from build123d import *

# Parameters (mm, degrees)
F1_DEPTH  = 25.4
F2_R      = 5.08
F3_T      = -6.35
F4_R      = 3.175
F5_DEPTH  = 38.1
F8_DEPTH  = 87.2033022895
F9_R      = 3.175
F10_DEPTH = 87.2033022895
F11_R     = 2.54
F12_DEPTH = 38.1


# Not quite as in the source:
# - the program builds the solid bodies; features that only make, move or delete a surface that nothing else refers to are left out


with BuildPart() as f1:
    # F0 (on Top) → F1 (new body)
    with BuildSketch(Plane.XY):
        Polygon((-43.9940905122, -76.2), (43.9940905122, -76.2), (87.9881810245, 0), (43.9940905122, 76.2), (-43.9940905122, 76.2), (-87.9881810245, 0), align=None)
    extrude(amount=F1_DEPTH)

    # F2
    f2_edges = [f1.edges().sort_by_distance(p)[0] for p in [
        (-65.991136, -38.1, 25.4),
        (0, -76.2, 25.4),
        (65.991136, -38.1, 25.4),
        (65.991136, 38.1, 25.4),
        (0, 76.2, 25.4),
        (-65.991136, 38.1, 25.4),
        (43.994091, -76.2, 12.7),
        (87.988181, 0, 12.7),
        (-43.994091, -76.2, 12.7),
        (43.994091, 76.2, 12.7),
        (-43.994091, 76.2, 12.7),
        (-87.988181, 0, 12.7),
    ]]
    fillet(f2_edges, radius=F2_R)

    # F3
    f3_openings = [f1.faces().sort_by_distance(p)[0] for p in [
        (0, 0, 0),
    ]]
    offset(amount=F3_T, openings=f3_openings)

    # F4 (on Right) → F5 (join)
    with BuildSketch(Plane.YZ):
        with Locations((76.2, 0)):
            Circle(F4_R)
    extrude(amount=-F5_DEPTH)

    # F8 (cut, through all): a face of the model
    f8_faces = [f1.faces().sort_by_distance(p)[0] for p in [
        (0, 76.6491706172, -0.4491706172),
    ]]
    extrude(f8_faces, amount=F8_DEPTH, mode=Mode.SUBTRACT)

    # F9 (on face) → F10 (cut, through all)
    with BuildSketch(Plane.YZ):
        with Locations((76.2, 0)):
            Circle(F9_R)
    extrude(amount=F10_DEPTH, mode=Mode.SUBTRACT)

    # F11 (on face) → F12 (join)
    with BuildSketch(Plane.YZ):
        with Locations((76.2, 0)):
            Circle(F11_R)
    extrude(amount=F12_DEPTH)


solid = f1.part
The listing builds one solid part. Answer for the finished solid, in the listing's coordinates (mm). A direction names the side the tool comes from. Coordinates: 2 decimals unless noted, no trailing zeros. Write each loop counter-clockwise with the first axis right and the second up, starting at its lowest first coordinate (ties: lowest second). Pieces come first, ordered by that corner, then holes. Notation, with made-up numbers: (63.5, 21) - (70.5, 21) arc R15 ccw to (70.5, 42) - close; hole circle Ø10 at (4.5, -1). An arc over 180 degrees is marked (long way). Put each result on its own line as item: value.
1. A tool of negligible diameter and unlimited length cuts with its end or side. For faces 5 (the face through (0, 78, 2)), 6 (the face through (0.575, -74.751, 23.872)), from which of +Z, -Z, +X, -X, +Y, -Y can it reach the whole face along a straight path? Write none if from no direction.
Answer sheet:
face 5: +X
face 6: +Z, +X, -X, -Y
2. Flat-ended cylindrical pins translate along their axes: pin 1 Ø5.5 at (y, z) = (77, -1) entering from +X; pin 2 Ø5 at (x, y) = (-1.5, -4.5) entering from -Z; pin 3 Ø6 at (y, z) = (-28.5, 16) entering from +X. Find the tip coordinate at first contact, or state that the pin passes through.
Answer sheet:
pin 1: stops at x = 38.1
pin 2: stops at z = 19.05
pin 3: stops at x = 73.27
3. The part is cut by section B-B on z = 5.5. Give the vertices of the cut face in (x, y), plus the area to 3 significant figures.
Answer sheet:
outline: (-86.52, -2.54) - (-45.46, -73.66) arc R5.08 ccw to (-41.06, -76.2) - (41.06, -76.2) arc R5.08 ccw to (45.46, -73.66) - (86.52, -2.54) arc R5.08 ccw to (86.52, 2.54) - (45.46, 73.66) arc R5.08 ccw to (41.06, 76.2) - (-41.06, 76.2) arc R5.08 ccw to (-45.46, 73.66) - (-86.52, 2.54) arc R5.08 ccw to start; hole (-80.66, 0) - (-40.33, -69.85) - (40.33, -69.85) - (80.66, 0) - (40.33, 69.85) - (-40.33, 69.85) - close
area: 3,200 mm^2
4. The part is cut by section A-A on x = 25. Give the vertices of the cut face in (y, z) (3 decimals).
Answer sheet:
outline: (-76.2, 0) - (-69.85, 0) - (-69.85, 19.05) - (69.85, 19.05) - (69.85, 0) - (73.025, 0) arc R3.175 cw to (76.2, 3.175) - (76.2, 20.32) arc R5.08 ccw to (71.12, 25.4) - (-71.12, 25.4) arc R5.08 ccw to (-76.2, 20.32) - close; circle Ø5.08 at (76.2, 0)
5. Determine the mould class of faces 1 (the face through (-60.21, 35.41, 9.39)), 2 (the face through (38.1, 76, 0)), 3 (the face through (-0.575, 74.751, 23.872)), 4 (the face through (-60.77, -34.44, 9.39)) for opening direction X: pulls with the +X half, pulls with the -X half, needs draft (parallel to the pull), parting line crosses it, or undercut.
Answer sheet:
face 1: undercut
face 2: pulls with the +X half
face 3: needs draft
face 4: undercut
6. Find the intervals of material crossed by line 1 along Y through (x, z) = (-18, 7); line 2 along Y through (x, z) = (19.5, 2); line 3 along Z through (x, y) = (-18.5, 9), in increasing order. Write a range as from..to.
Answer sheet:
line 1: y = -76.2..-69.85, 69.85..76.2
line 2: y = -76.2..-69.85, 69.85..73.73, 74.63..77.77
line 3: z = 19.05..25.4
